Print and shaded views of the part. All mm, measured from the part's lowest x, y and z. A direction names the side the tool comes from. Give positions to 0.01 mm unless a question says otherwise; leave off trailing zeros. Write each loop counter-clockwise with the first axis right and the second up, starting at its lowest first coordinate (ties: lowest second). Pieces come first, ordered by that corner, then holes. Notation, with made-up numbers: (24.25, -27) -> (64.25, -27) arc R34 ccw to (64.25, 11) -> close; hole circle Ø11 at (29, -7.75). An arc over 180 degrees is marked (long way). Put each result on its own line as item: value.
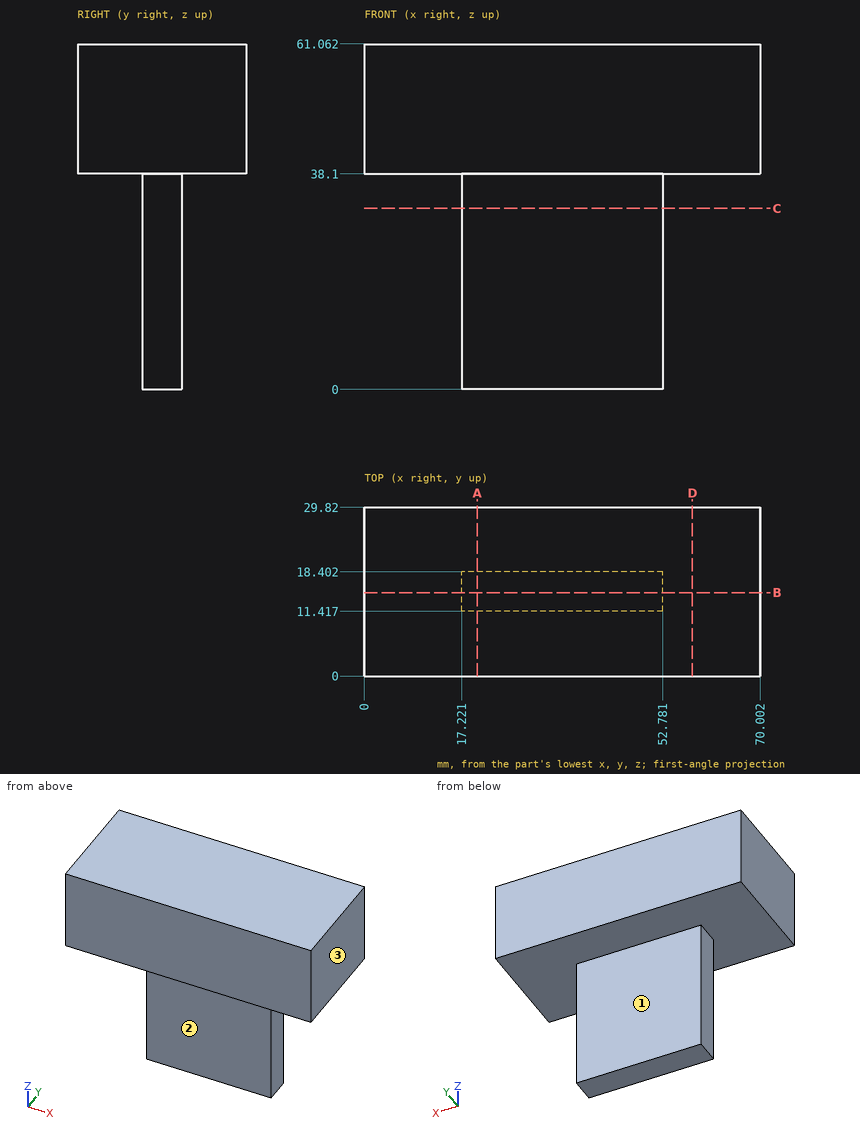
1) Wall check: L1, parallel to Z at x = 24.5, y = 3; L2, parallel to Y at x = 28, z = 25; L3, parallel to X at y = 17.5, z = 32. Give the ranges that are in metal, low to high.
Filled sheet:
L1: 38.1 to 61.06
L2: 11.42 to 18.4
L3: 17.22 to 52.78
2) Slice it at B-B (y = 14.75). Write the cut outline in (x, z), plus the area to 3 significant figures.
Filled sheet:
outline: (0, 38.1) -> (17.22, 38.1) -> (17.22, 0) -> (52.78, 0) -> (52.78, 38.1) -> (70, 38.1) -> (70, 61.06) -> (0, 61.06) -> close
area: 2,960 mm2
3) Slice it at A-A (x = 20). Write the cut outline in (y, z).
Filled sheet:
outline: (0, 38.1) -> (11.42, 38.1) -> (11.42, 0) -> (18.4, 0) -> (18.4, 38.1) -> (29.82, 38.1) -> (29.82, 61.06) -> (0, 61.06) -> close
4) Slice it at D-D (x = 58). Write the cut outline in (y, z).
Filled sheet:
outline: (0, 38.1) -> (29.82, 38.1) -> (29.82, 61.06) -> (0, 61.06) -> close
5) Slice it at C-C (z = 32). Write the cut outline in (x, y), plus the area to 3 significant figures.
Filled sheet:
outline: (17.22, 11.42) -> (52.78, 11.42) -> (52.78, 18.4) -> (17.22, 18.4) -> close
area: 248 mm2
6) Tool access for the marked faces 1, 2 and 3: list every direction of +Z, -Z, +X, -X, +Y, -Y with a clear straight run to the whole face (end or side of a thin tool).
Filled sheet:
face 1: -Z, +X, -X, +Y
face 2: -Z, +X, -X, -Y
face 3: +Z, -Z, +X, +Y, -Y
7) Pin check, flat tips, straight feed: pin 1 (2 mm diameter, centred on x = 33, y = 21.5, fed in from -Z); pin 2 (3.5 mm diameter, centred on y = 14.5, z = 15, fed in from +X); pin 3 (2 mm diameter, centred on y = 16, z = 9.5, fed in from -X); pin 4 (6 mm diameter, centred on y = 6, z = 19, fed in from -X). Stop position of each tip, or through.
Filled sheet:
pin 1: z = 38.1
pin 2: x = 52.78
pin 3: x = 17.22
pin 4: through
